Part model, mm, in its own coordinate system. Round coordinates to 2 decimals unless told otherwise and drop trailing zeros. Loops run counter-clockwise (first coordinate to the right, second up) from the corner with the lowest first, then second, coordinate; pieces in that order, holes last. Notation, with made-up numbers: M 45,79 L 94,79 A29 cw 94,103 Z; hole C -10.5,57 d9. An arc over 180 degrees is marked long. Put each result on its own line as item: value. Start each with the question number.
Autodesk Inventor part; units mm, degrees
ref_plane "YZ Plane" through (0, 0, 0) normal (1, 0, 0) x (0, 1, 0)
ref_plane "XZ Plane" through (0, 0, 0) normal (0, 1, 0) x (-1, 0, 0)
ref_plane "XY Plane" through (0, 0, 0) normal (0, 0, 1) x (1, 0, 0)
sketch "Sketch1" plane through (0, 0, 0) normal (1, 0, 0) x (0, 1, 0)
  line L0 (95.25, 812.8) -> (44.45, 812.8) construction
  line L1 (44.45, 812.8) -> (44.45, 0) construction
  line L2 (44.45, 0) -> (95.25, 0) construction
  line L3 (95.25, 0) -> (95.25, 812.8) construction
  line L4 (95.25, 0) -> (44.45, 0) construction
  line L5 (44.45, 25.4) -> (95.25, 25.4) construction
  circle A0 centre (190.5, 0) radius 50.8 construction
  circle A1 centre (95.25, 279.4) radius 25.4 construction
  circle A2 centre (274.9493, 279.9916) radius 9.525
  circle A3 centre (274.9493, 279.9916) radius 25.4 construction
  circle A4 centre (274.9493, 279.9916) radius 31.75 construction
  circle A5 centre (299.4838, 286.5656) radius 2.4892
  circle A6 centre (292.9098, 297.9521) radius 2.4892
  circle A7 centre (281.5233, 304.5261) radius 2.4892
  circle A8 centre (268.3753, 304.5261) radius 2.4892
  circle A9 centre (256.9887, 297.9521) radius 2.4892
  circle A10 centre (250.4147, 286.5656) radius 2.4892 construction
  circle A11 centre (250.4147, 273.4176) radius 2.4892 construction
  circle A12 centre (256.9887, 262.0311) radius 2.4892
  circle A13 centre (268.3753, 255.4571) radius 2.4892
  circle A14 centre (281.5233, 255.4571) radius 2.4892 construction
  circle A15 centre (292.9098, 262.0311) radius 2.4892 construction
  circle A16 centre (299.4838, 273.4176) radius 2.4892
  circle A17 centre (609.6, 438.15) radius 50.8 construction
  circle A18 centre (274.9493, 279.9916) radius 30.48 construction
  circle A19 centre (587.8333, 365.125) radius 25.4 construction
  circle A20 centre (587.8333, 511.175) radius 25.4 construction
  line L6 (587.8333, 485.775) -> (587.8333, 390.525) construction
  circle A21 centre (490.3356, 512.7625) radius 14.351
  circle A22 centre (392.825, 512.7625) radius 14.351
  circle A23 centre (490.3356, 363.5375) radius 14.351
  line L7 (587.8333, 511.175) -> (490.3356, 512.7625) construction
  line L8 (587.8333, 365.125) -> (490.3356, 363.5375) construction
  circle A24 centre (490.3356, 512.7625) radius 25.4 construction
  circle A25 centre (490.3356, 363.5375) radius 25.4 construction
  line L9 (490.3356, 487.3625) -> (490.3356, 388.9375) construction
  circle A26 centre (392.825, 512.7625) radius 25.4 construction
  circle A27 centre (392.825, 363.5375) radius 25.4 construction
  circle A28 centre (392.825, 363.5375) radius 14.351
  line L10 (490.3356, 512.7625) -> (392.825, 512.7625) construction
  line L11 (490.3356, 363.5375) -> (392.825, 363.5375) construction
  line L12 (392.825, 487.3625) -> (392.825, 388.9375) construction
  circle A29 centre (295.3189, 511.8309) radius 25.4 construction
  circle A30 centre (295.3189, 362.6059) radius 25.4 construction
  circle A31 centre (203.1597, 479.9719) radius 25.4 construction
  circle A32 centre (295.3189, 511.8309) radius 14.351
  circle A33 centre (295.3189, 362.6059) radius 14.351
  circle A34 centre (203.1597, 479.9719) radius 14.351
  line L13 (392.825, 512.7625) -> (295.3189, 511.8309) construction
  line L14 (392.825, 363.5375) -> (295.3189, 362.6059) construction
  line L15 (295.3189, 486.4309) -> (295.3189, 388.0059) construction
  line L16 (295.3189, 511.8309) -> (203.1597, 479.9719) construction
  circle A35 centre (123.1487, 424.2353) radius 25.4 construction
  circle A36 centre (123.1487, 424.2353) radius 14.351
  line L17 (203.1597, 479.9719) -> (123.1487, 424.2353) construction
  circle A37 centre (95.25, 279.4) radius 14.351
  line L18 (609.6, 355.6) -> (44.45, 355.6) construction
  line L19 (44.45, 355.6) -> (44.45, 330.2) construction
  line L20 (44.45, 330.2) -> (609.6, 330.2) construction
  line L21 (609.6, 330.2) -> (609.6, 355.6) construction
  line L22 (95.25, 241.3) -> (44.45, 241.3) construction
  line L23 (44.45, 241.3) -> (44.45, 215.9) construction
  line L24 (44.45, 215.9) -> (95.25, 215.9) construction
  line L25 (95.25, 215.9) -> (95.25, 241.3) construction
  circle A38 centre (244.475, 279.4) radius 25.4 construction
  circle A39 centre (244.475, 279.4) radius 14.351
  line L26 (218.8463, 459.9947) -> (279.6322, 382.5831) construction
  circle A40 centre (274.9493, 279.9916) radius 8.89 construction
  circle A41 centre (288.401, 252.6405) radius 21.59 construction
  circle A42 centre (244.475, 279.4) radius 21.59 construction
  circle A43 centre (288.401, 252.6405) radius 14.351
  circle A44 centre (587.8333, 511.175) radius 14.351
  circle A45 centre (587.8333, 365.125) radius 14.351
  line L27 (95.25, 647.7) -> (609.6, 647.7) construction
  line L28 (609.6, 647.7) -> (609.6, 622.3) construction
  line L29 (609.6, 622.3) -> (95.25, 622.3) construction
  line L30 (95.25, 622.3) -> (95.25, 647.7) construction
  circle A46 centre (600.5333, 552.45) radius 3.2639
  circle A47 centre (600.5333, 552.45) radius 6.35 construction
  circle A48 centre (600.5333, 336.55) radius 3.2639
  circle A49 centre (600.5333, 336.55) radius 6.35 construction
  circle A50 centre (114.3, 552.45) radius 3.2639
  circle A51 centre (114.3, 552.45) radius 6.35 construction
  line L31 (595.3031, 535.4518) -> (598.6659, 546.3808) construction
  circle A52 centre (63.5, 264.8503) radius 3.2639
  circle A53 centre (63.5, 264.8503) radius 6.35 construction
  line L32 (337.9424, 330.2) -> (600.5333, 330.2)
  circle A54 centre (288.401, 252.6405) radius 24.13 construction
  circle A55 centre (244.475, 279.4) radius 24.13 construction
  line L33 (72.1591, 268.8184) -> (69.2727, 267.4957) construction
  line L34 (609.6, 342.9) -> (44.45, 342.9) construction
  circle A56 centre (288.401, 252.6405) radius 19.05 construction
  line L35 (265.0822, 266.8462) -> (267.7937, 265.1944) construction
  circle A57 centre (318.8924, 273.2978) radius 3.2639
  circle A58 centre (253.4257, 241.1003) radius 3.2639
  line L36 (95.25, 558.8) -> (44.45, 558.8) construction
  line L37 (44.45, 558.8) -> (44.45, 533.4) construction
  line L38 (44.45, 533.4) -> (95.25, 533.4) construction
  line L39 (95.25, 533.4) -> (95.25, 558.8) construction
  line L40 (114.3, 558.8) -> (600.5333, 558.8)
  line L41 (108.0468, 553.5545) -> (57.2468, 265.9549)
  line L42 (285.1949, 228.7245) -> (62.6563, 258.5566)
  circle A59 centre (318.8924, 273.2978) radius 6.35 construction
  circle A60 centre (253.4257, 241.1003) radius 6.35 construction
  arc A61 (114.3, 558.8) -> (108.0468, 553.5545) centre (114.3, 552.45) ccw
  arc A62 (57.2468, 265.9549) -> (62.6563, 258.5566) centre (63.5, 264.8503) ccw
  line L43 (312.6148, 274.2541) -> (306.3372, 275.2103) construction
  line L44 (313.6352, 269.7362) -> (308.3781, 266.1746) construction
  line L45 (259.4559, 243.09) -> (265.4861, 245.0797) construction
  line L46 (256.5005, 246.6562) -> (259.5753, 252.2121) construction
  line L47 (325.2424, 317.5) -> (325.2424, 273.2978)
  arc A63 (337.9424, 330.2) -> (325.2424, 317.5) centre (337.9424, 317.5) ccw
  line L48 (324.5494, 270.4133) -> (309.8976, 241.6792)
  arc A64 (324.5494, 270.4133) -> (325.2424, 273.2978) centre (318.8924, 273.2978) ccw
  arc A65 (285.1949, 228.7245) -> (309.8976, 241.6792) centre (288.401, 252.6405) ccw
  circle A66 centre (431.8, 342.9) radius 3.2639
  circle A67 centre (457.2, 342.9) radius 3.2639
  circle A68 centre (520.7, 342.9) radius 3.2639
  circle A69 centre (546.1, 342.9) radius 3.2639
  line L49 (606.8833, 552.45) -> (606.8833, 336.55)
  arc A70 (606.8833, 552.45) -> (600.5333, 558.8) centre (600.5333, 552.45) ccw
  arc A71 (600.5333, 330.2) -> (606.8833, 336.55) centre (600.5333, 336.55) ccw
  circle A72 centre (184.15, 304.8) radius 3.2639
  circle A73 centre (158.75, 304.8) radius 3.2639
  circle A74 centre (133.35, 304.8) radius 3.2639
  circle A75 centre (133.35, 279.4) radius 3.2639
  circle A76 centre (158.75, 279.4) radius 3.2639
  circle A77 centre (184.15, 279.4) radius 3.2639
  circle A78 centre (502.1083, 584.2) radius 3.2639
  circle A79 centre (197.3083, 584.2) radius 3.2639
  circle A80 centre (349.7083, 584.2) radius 3.2639
  circle A81 centre (502.1083, 584.2) radius 12.7 construction
  circle A82 centre (197.3083, 584.2) radius 12.7 construction
  line L50 (556.0833, 558.8) -> (509.8384, 594.2765)
  line L51 (191.9353, 595.7074) -> (111.6135, 558.2037)
  line L52 (197.3083, 596.9) -> (502.1083, 596.9)
  arc A83 (197.3083, 596.9) -> (191.9353, 595.7074) centre (197.3083, 584.2) ccw
  arc A84 (509.8384, 594.2765) -> (502.1083, 596.9) centre (502.1083, 584.2) ccw
  point P0 (0, 0)
  point P1 (274.0548, 252.2687)
  point P2 (274.7516, 257.073)
  point P3 (251.6966, 266.9984)
  point P4 (254.3358, 268.9733)
  point P5 (241.139, 234.6303)
  point P6 (100.4185, 253.4945)
  dimension "d9" = 50.8
  dimension "d14" = 50.8
  dimension "d38" = 50.8
  dimension "d53" = 50.8
  dimension "d1" = 812.8
  dimension "d2" = 44.45
  dimension "d4" = 25.4
  dimension "d5" = 101.6
  dimension "d6" = 95.25
  dimension "d8" = 50.8
  dimension "d15" = 63.5
  dimension "d21" = 19.05
  dimension "d26" = 360
  dimension "d28" = 4.9784
  dimension "d29" = 438.15
  dimension "d30" = 514.35
  dimension "d36" = 60.96
  dimension "d39" = 50.8
  dimension "d41" = 95.25
  dimension "d45" = 28.702
  dimension "d47" = 97.5106
  dimension "d48" = 98.425
  dimension "d56" = 25.4
  dimension "d73" = 50.8
  dimension "d74" = 25.4
  dimension "d75" = 215.9
  dimension "d78" = 279.4
  dimension "d80" = 149.225
  dimension "d81" = 97.5106
  dimension "d82" = 147.4978
  dimension "d83" = 17.78
  dimension "d85" = 43.18
  dimension "d92" = 330.2
  dimension "d100" = 514.35
  dimension "d107" = 25.4
  dimension "d108" = 514.35
  dimension "d109" = 266.7
  dimension "d115" = 6.5278
  dimension "d116" = 12.7
  dimension "d122" = 2.54
  dimension "d123" = 2.54
  dimension "d128" = 3.175
  dimension "d133" = 38.1
  dimension "d134" = 3.175
  dimension "d135" = 194.9958
  dimension "d136" = 6.5278
  dimension "d137" = 25.4
  dimension "d138" = 533.4
  dimension "d139" = 19.05
  dimension "d140" = 19.05
  dimension "d141" = 12.7
  dimension "d142" = 6.35
  dimension "d143" = 12.7
  dimension "d144" = 43.18
  dimension "d149" = 25.4
  dimension "d151" = 6.5278
  dimension "d157" = 25.4
  dimension "d158" = 63.5
  dimension "d159" = 12.7
  dimension "d161" = 11.4347
  dimension "d163" = 44.45
  dimension "d164" = 38.1
  dimension "d166" = 336.55
  dimension "d167" = 25.4
  dimension "d168" = 6.5278
  dimension "d169" = 25.4
  dimension "d170" = 25.4
  dimension "d173" = 25.4
extrude "Extrusion2" add sketch "Sketch1" along normal blind 6.35 contours A9 | A16 | A63 L47 A64 L48 A65 L42 A62 L41 A61 L40 A70 L49 A71 L32 | L40 A61 L51 A83 L52 A84 L50
properties part number "sketchers" material "Polycarbonate, Clear"
1. Drop flat-ended pins along their axis: pin 1 (1 mm diameter, centred on x = 2, y = 294, fed in from -Z); pin 2 (3 mm diameter, centred on y = 504.5, z = 493, fed in from -X); pin 3 (15 mm diameter, centred on y = 274.95, z = 279.99, fed in from +X); pin 4 (2 mm diameter, centred on x = 1.5, y = 115, fed in from -Z). Give the stop position or say it passes through.
2. Cut at A-A, the plane x = 2. Give the number of separate pieces and of enclosed holes in the cut face, and give its area (3 significant figures).
3. Cut at B-B, the plane z = 571.5. Give the cut face in (x, y), and give its area (3 significant figures).
4. Wall check: L1, parallel to Z at x = 5, y = 160; L2, parallel to Y at x = 2.5, z = 552.45; L3, parallel to Y at x = 2.75, z = 304.8. Give the ranges that are in metal, low to high.
5. Mould opens along Y. For faces 1 (the flat face through (3.131, 533.285, 576.29)), 2 (the flat face through (3.131, 83.002, 411.768)), 3 (the cylindrical face through (3.13, 257.73, 284.9)), 4 (the flat face through (0, 328, 415)) say: released by +Y, released by -Y, zero draft, split by the parting line, or undercut.
Results list:
1. pin 1: stops at z = 229.06
1. pin 2: stops at x = 0
1. pin 3: passes through
1. pin 4: stops at z = 251.41
2. separate pieces: 1
2. enclosed holes: 39
2. area: 146,000 mm^2
3. outline: M 0,140.09 L 6.35,140.09 L 6.35,539.53 L 0,539.53 Z
3. area: 2,540 mm^2
4. L1: z = 245.51 to 276.38, 282.42 to 301.78, 307.82 to 580.8
4. L2: y = 107.85 to 111.04, 117.56 to 597.27, 603.8 to 606.88
4. L3: y = 64.11 to 130.09, 136.61 to 155.49, 162.01 to 180.89, 187.41 to 265.9, 270.85 to 279.05, 284 to 325.24
5. face 1: released by +Y
5. face 2: released by -Y
5. face 3: undercut
5. face 4: zero draft
